Here's the drawing with two shaded views (mm, measured from the low corner). I have some questions. Give positions to 0.01 mm unless a question says otherwise; leave off trailing zeros. Loops run counter-clockwise (first coordinate to the right, second up) from the corner with the lowest first, then second, coordinate; pieces in that order, holes last. Notation, with made-up numbers: (45, -24.5) - (104, -24.5) arc R23 cw to (104, -10.5) - close; hole circle Ø10 at (84.25, 75.25). An arc over 180 degrees is marked (long way). Answer as a JSON object with one key per item and string values. Group by question number.
Item 1: Suppose I cut it at A-A on x = 36. Write out the boundary of the cut face in (y, z).
Item 2: Suppose I cut it at D-D on x = 4.9. Write out the boundary of the cut face in (y, z), and give its area (3 significant figures).
Item 3: Suppose I cut it at B-B on y = 10. Write out the boundary of the cut face in (x, z).
Item 4: Suppose I cut it at C-C on z = 0.8. Write out the boundary of the cut face in (x, y).
Item 5: Will this pin go through, and if not, where does the flat tip stop? pin 1 (3 mm diameter, centred on x = 4.9, y = 10, fed in from +Z).
Item 6: Please list where these lines run through material, in increasing order: L1, parallel to Y at x = 36, z = 0.4; L2, parallel to Y at x = 67.1, z = 0.4; L3, parallel to X at y = 12, z = 0.5.
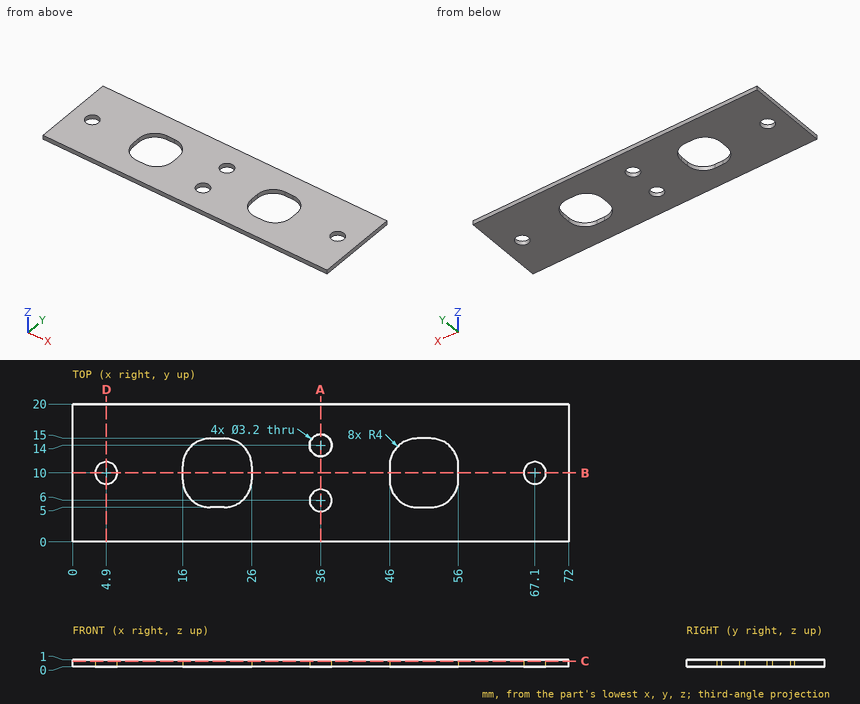
Worked out:
{
 "1": {"outline": "(0, 0) - (4.4, 0) - (4.4, 1) - (0, 1) - close; (7.6, 0) - (12.4, 0) - (12.4, 1) - (7.6, 1) - close; (15.6, 0) - (20, 0) - (20, 1) - (15.6, 1) - close"},
 "2": {"outline": "(0, 0) - (8.4, 0) - (8.4, 1) - (0, 1) - close; (11.6, 0) - (20, 0) - (20, 1) - (11.6, 1) - close", "area": "16.8 mm2"},
 "3": {"outline": "(0, 0) - (3.3, 0) - (3.3, 1) - (0, 1) - close; (6.5, 0) - (16, 0) - (16, 1) - (6.5, 1) - close; (26, 0) - (46, 0) - (46, 1) - (26, 1) - close; (56, 0) - (65.5, 0) - (65.5, 1) - (56, 1) - close; (68.7, 0) - (72, 0) - (72, 1) - (68.7, 1) - close"},
 "4": {"outline": "(0, 0) - (72, 0) - (72, 20) - (0, 20) - close; hole circle Ø3.2 at (4.9, 10); hole (16, 9) arc R4 ccw to (20, 5) - (22, 5) arc R4 ccw to (26, 9) - (26, 11) arc R4 ccw to (22, 15) - (20, 15) arc R4 ccw to (16, 11) - close; hole circle Ø3.2 at (36, 6); hole circle Ø3.2 at (36, 14); hole (46, 9) arc R4 ccw to (50, 5) - (52, 5) arc R4 ccw to (56, 9) - (56, 11) arc R4 ccw to (52, 15) - (50, 15) arc R4 ccw to (46, 11) - close; hole circle Ø3.2 at (67.1, 10)"},
 "5": {"pin 1": "passes through"},
 "6": {"L1": "y = 0 to 4.4, 7.6 to 12.4, 15.6 to 20", "L2": "y = 0 to 8.4, 11.6 to 20", "L3": "x = 0 to 16.13, 25.87 to 46.13, 55.87 to 72"}
}
